Geometry check sheet. Reference: the model listing, model coordinates, mm. A direction names the side the tool comes from. Round coordinates to 2 decimals unless told otherwise and drop trailing zeros. Order: outer loops, then holes, each group sorted by start corner. A loop starts at its lowest first (then second) coordinate and runs counter-clockwise, first axis right, second up.
(1) Set-up check for faces 4 (the face through (3, 1, 1)), 5 (the face through (-3, 1, 1)): record each of +Z, -Z, +X, -X, +Y, -Y from which the full face is reachable in a straight line by a thin tool's end or side.
(2) Cross-section at C-C on z = 1.3. Enter the section's corners in (x, y).
(3) Cross-section at D-D on x = 0. Enter the section's corners in (y, z).
(4) Cross-section at A-A on y = 20. Enter the section's corners in (x, z).
(5) Draft check along X on faces 1 (the face through (-2.43, 22.4, 1.01)), 2 (the face through (2, -14, 0)), 3 (the face through (6.66, -47.96, 0.99)). Enter one of: pulls with the +X half, pulls with the -X half, needs draft (parallel to the pull), parting line crosses it, or undercut.
(6) Cross-section at B-B on x = 8.5. Enter the section's corners in (y, z), and give its area (3 significant figures).
(7) Gauge pin test, flat end, axial feed: P1, Ø1.8, axis at x = 7.76, y = -48.98, coming from the -Z side. Record the tip position at first contact, or that the pin passes through.
(8) Thickness scan on L1, parallel to X at y = 3, z = 1; L2, parallel to X at y = -35, z = 0.7. Record the ranges inside material, lowest first.
from build123d import *

# Parameters (mm, degrees)
ESQUISSE2_R        = 1.5
BOSS_EXTRU_3_DEPTH = 2
CONG_3_R           = 2


with BuildPart() as part:
    # Esquisse2 → Boss.-Extru.3 (new body)
    with BuildSketch(Plane.XY):
        Polygon((-3, 23), (-3, -20.394957493), (5.64325101, -52.652009403), (11.438805967, -51.099095132), (3, -19.605042507), (3, 23), align=None)
        with Locations((7.764571353, -48.977774789)):
            Circle(ESQUISSE2_R, mode=Mode.SUBTRACT)
        with Locations((0, -20)):
            Circle(ESQUISSE2_R, mode=Mode.SUBTRACT)
        with Locations((0, 20)):
            Circle(ESQUISSE2_R, mode=Mode.SUBTRACT)
    extrude(amount=BOSS_EXTRU_3_DEPTH)

    # Congé3
    cong_3_edges = [part.edges().sort_by_distance(p)[0] for p in [
        (-3, -20.394957493, 1),
        (-3, 23, 1),
        (3, 23, 1),
        (3, -19.605042507, 1),
        (11.438805967, -51.099095132, 1),
        (5.64325101, -52.652009403, 1),
    ]]
    fillet(cong_3_edges, radius=CONG_3_R)


solid = part.part
Found:
1. face 4: +Z, -Z, +X, +Y
1. face 5: +Z, -Z, -X, +Y, -Y
2. outline: (-3, -20.13) arc R2 ccw to (-2.93, -20.65) - (5.13, -50.72) arc R2 ccw to (7.58, -52.13) - (9.51, -51.62) arc R2 ccw to (10.92, -49.17) - (3.07, -19.86) arc R2 cw to (3, -19.34) - (3, 21) arc R2 ccw to (1, 23) - (-1, 23) arc R2 ccw to (-3, 21) - close; hole circle Ø3 at (0, -20); hole circle Ø3 at (0, 20); hole circle Ø3 at (7.76, -48.98)
3. outline: (-31.59, 0) - (-21.5, 0) - (-21.5, 2) - (-31.59, 2) - close; (-18.5, 0) - (18.5, 0) - (18.5, 2) - (-18.5, 2) - close; (21.5, 0) - (23, 0) - (23, 2) - (21.5, 2) - close
4. outline: (-3, 0) - (-1.5, 0) - (-1.5, 2) - (-3, 2) - close; (1.5, 0) - (3, 0) - (3, 2) - (1.5, 2) - close
5. face 1: pulls with the -X half
5. face 2: needs draft
5. face 3: undercut
6. outline: (-51.89, 0) - (-50.29, 0) - (-50.29, 2) - (-51.89, 2) - close; (-47.67, 0) - (-40.13, 0) - (-40.13, 2) - (-47.67, 2) - close
6. area: 18.3 mm2
7. P1: passes through
8. L1: x = -3 to 3
8. L2: x = 0.91 to 7.13
